```python
from build123d import *

# Parameters (mm, degrees)
ESQUISSE1_R        = 23.5
ESQUISSE1_R_2      = 15
BOSS_EXTRU_1_DEPTH = 3.14
ESQUISSE2_R        = 2.75
CONG_1_R           = 0.6


with BuildPart() as part:
    # Esquisse1 → Boss.-Extru.1 (new body)
    with BuildSketch(Plane.XY):
        Circle(ESQUISSE1_R)
        Circle(ESQUISSE1_R_2, mode=Mode.SUBTRACT)
    extrude(amount=BOSS_EXTRU_1_DEPTH)

    # Esquisse2 → Enlèvement de matière-Révolution1 (revolve, cut)
    with BuildSketch(Plane(origin=(0, 0, 0), x_dir=(1, 0, 0), z_dir=(0, 1, 0)), mode=Mode.PRIVATE) as enl_vement_de_mati_re_r_volution1_sk:
        with Locations((19.75, -5.5)):
            Circle(ESQUISSE2_R)
    revolve(enl_vement_de_mati_re_r_volution1_sk.sketch.rotate(Axis((0, 0, 0), (0, 0, 1)), 180), axis=Axis((0, 0, 0), (0, 0, 1)), mode=Mode.SUBTRACT)

    # Congé1
    cong_1_edges = [part.edges().sort_by_distance(p)[0] for p in [
        (-23.5, 0, 0),
        (-23.5, 0, 3.14),
        (-15, 0, 0),
        (-15, 0, 3.14),
    ]]
    fillet(cong_1_edges, radius=CONG_1_R)


solid = part.part
```
Can you work these out from the model? Positions are in its coordinate system, mm. Round coordinates to 2 decimals unless told otherwise and drop trailing zeros. Loops run counter-clockwise (first coordinate to the right, second up) from the corner with the lowest first, then second, coordinate; pieces in that order, holes last.
Item 1: Suppose I cut it at B-B, the plane z = 1.2. Write out the boundary of the cut face in (x, y), then the cut area to 3 significant figures.
Item 2: Will this pin go through, and if not, where does the flat tip stop? pin 1 Ø1 at (x, z) = (-3.5, 1) entering from -Y.
Item 3: Suppose I cut it at A-A, the plane x = 0. Write out the boundary of the cut face in (y, z), then the cut area to 3 significant figures.
Item 4: Please list where these lines run through material, in increasing order: L1, parallel to Y at x = 0, z = 1.35; L2, parallel to X at y = 10, z = 0.5; L3, parallel to X at y = -7, z = 0.85.
Item 5: If we mould it in two halves opening along Y, with no side actions, what happens to faces 1 (the cylindrical face through (-14.985, 0.66, 1.556)), 2 (the flat face through (20.25, -6.68, 3.14)), 3 (the cylindrical face through (22.4, 7.1, 1.6))? For each: +Y half, -Y half, draft (parallel to the pull), parting line (faces both ways), or undercut.
Reported:
1. outline: circle Ø47 at (0, 0); hole circle Ø30 at (0, 0)
1. area: 1,030 mm2
2. pin 1: stops at y = -23.31
3. outline: (-23.5, 0.6) arc R0.6 ccw to (-22.9, 0) - (-15.6, 0) arc R0.6 ccw to (-15, 0.6) - (-15, 2.54) arc R0.6 ccw to (-15.6, 3.14) - (-18.34, 3.14) arc R2.75 cw to (-21.16, 3.14) - (-22.9, 3.14) arc R0.6 ccw to (-23.5, 2.54) - close; (15, 0.6) arc R0.6 ccw to (15.6, 0) - (22.9, 0) arc R0.6 ccw to (23.5, 0.6) - (23.5, 2.54) arc R0.6 ccw to (22.9, 3.14) - (21.16, 3.14) arc R2.75 cw to (18.34, 3.14) - (15.6, 3.14) arc R0.6 ccw to (15, 2.54) - close
3. area: 51.3 mm2
4. L1: y = -23.5 to -15, 15 to 23.5
4. L2: x = -21.26 to -11.19, 11.19 to 21.26
4. L3: x = -22.43 to -13.27, 13.27 to 22.43
5. face 1: undercut
5. face 2: draft
5. face 3: parting line
